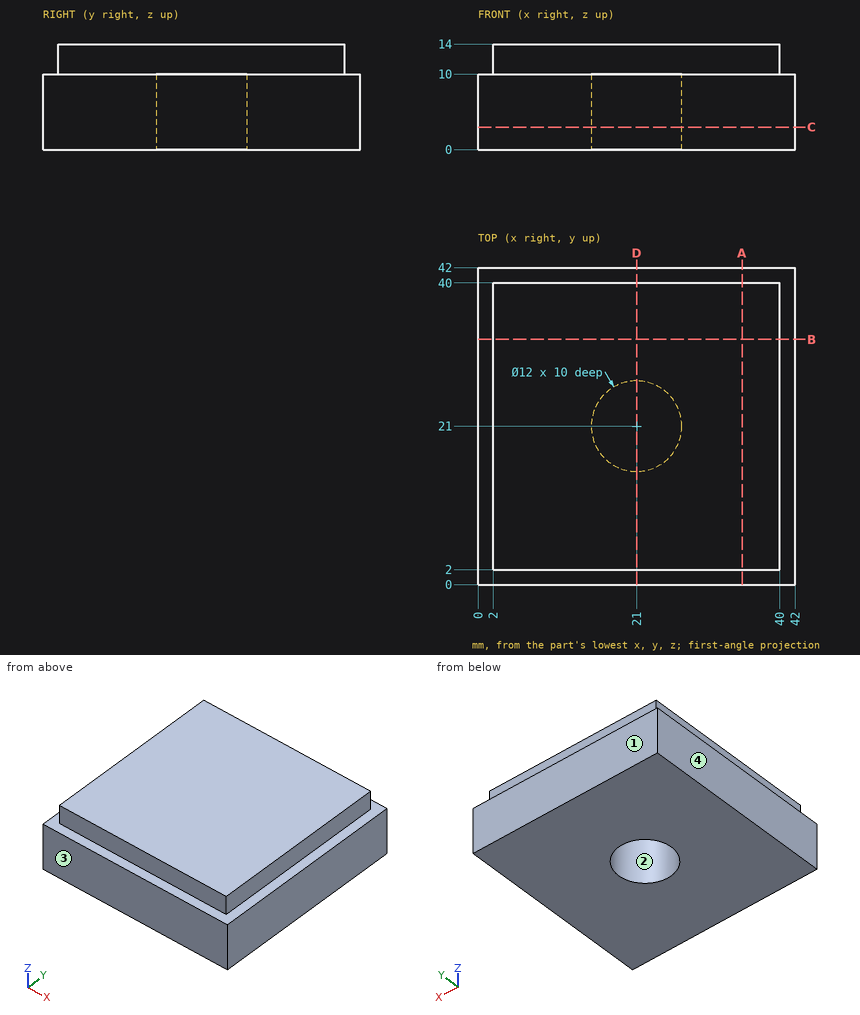
Drawing for the job (mm, zero at the part's lowest x, y, z). Give positions to 0.01 mm unless a question says otherwise; leave off trailing zeros. Loops run counter-clockwise (first coordinate to the right, second up) from the corner with the lowest first, then second, coordinate; pieces in that order, holes last. Notation, with made-up numbers: M 57,19.5 L 79,19.5 A23 ccw 79,51.5 Z; hole C 33,49 d6. An arc over 180 degrees is marked long. One line per question, with ' | ' between items. Start each with the question number.
1. Two-plate mould, pull along Y, no slides. Class the marked faces 1, 2, 3 and 4: pulls with the +Y half, pulls with the -Y half, needs draft (parallel to the pull), parting line crosses it, or undercut.
2. Flat gauge pins, fed straight in: pin 1 (3 mm diameter, centred on y = 29, z = 13, fed in from -X); pin 2 (1.2 mm diameter, centred on y = 22, z = 12.5, fed in from +X); pin 3 (2 mm diameter, centred on x = 25, z = 13, fed in from -Y). Where does each tip first touch, or does it go through?
3. Saw through at C-C on z = 3. Give the cut face in (x, y), plus the area to 3 significant figures.
4. Saw through at A-A on x = 35. Give the cut face in (y, z), plus the area to 3 significant figures.
5. Probe L1, parallel to Y at x = 21, z = 5.75; L2, parallel to Y at x = 19.5, z = 4.25; L3, parallel to X at y = 32, z = 11. List the from-to ranges inside material, lowest first. Write a range as from..to.
6. Saw through at D-D on x = 21. Give the cut face in (y, z), plus the area to 3 significant figures.
Result sheet:
1) face 1: pulls with the +Y half | face 2: undercut | face 3: pulls with the -Y half | face 4: needs draft
2) pin 1: stops at x = 2 | pin 2: stops at x = 40 | pin 3: stops at y = 2
3) outline: M 0,0 L 42,0 L 42,42 L 0,42 Z; hole C 21,21 d12 | area: 1,650 mm^2
4) outline: M 0,0 L 42,0 L 42,10 L 40,10 L 40,14 L 2,14 L 2,10 L 0,10 Z | area: 572 mm^2
5) L1: y = 0..15, 27..42 | L2: y = 0..15.19, 26.81..42 | L3: x = 2..40
6) outline: M 0,0 L 15,0 L 15,10 L 27,10 L 27,0 L 42,0 L 42,10 L 40,10 L 40,14 L 2,14 L 2,10 L 0,10 Z | area: 452 mm^2
